Could you check a few things on this model? Use its own coordinates, in mm. A direction names the side the tool comes from. Round coordinates to 2 decimals unless told otherwise and drop trailing zeros. Loops run counter-clockwise (first coordinate to the right, second up) from the corner with the lowest first, then second, coordinate; pieces in that order, holes last. Notation, with made-up numbers: (-37, 87) - (19, 87) arc R14 ccw to (19, 97) - close; hole circle Ø3 at (-18, 61). An arc over 180 degrees is marked (long way). Answer as CSV lines item,"result". Start each with the question number.
1) Suppose I cut it at B-B, the plane z = 13.5. Write out the boundary of the cut face in (x, y), then the cut area to 3 significant figures.
2) We'd pull the mould along Z, two halves only. Please class faces 1 (the face through (61, 20, 26.5)), 2 (the face through (15.175, 68.335, 22.204)), 3 (the face through (66.94, 0.09, 5.8)): pulls with the +Z half, pulls with the -Z half, needs draft (parallel to the pull), parting line crosses it, or undercut.
3) Which directions (+Z, -Z, +X, -X, +Y, -Y) give clear straight access to the entire face, cutting with the end or side of a thin tool? Please do faces 4 (the face through (52, 46, 9)), 5 (the face through (15.175, 68.335, 5.704)).
4) Please list where these lines run through material, in increasing order: line 1 along Z through (x, y) = (31, -62); line 2 along Y through (x, z) = (0, 12.5); line 3 along Y through (x, z) = (-14.5, 7).
5) Suppose I cut it at A-A, the plane x = 0. Write out the boundary of the cut face in (y, z), then the cut area to 3 significant figures.
6) I'm going to push flat-ended pins straight in: pin 1 Ø6 at (y, z) = (54.5, 7.5) entering from -X; pin 2 Ø1 at (y, z) = (50, 9) entering from +X; pin 3 Ø12 at (x, z) = (-53, 14.5) entering from -Y. Where does each tip first touch, or does it pass through?
```python
from build123d import *

# Parameters (mm, degrees)
SKETCH2_R           = 2.2
GRUB_KEY_HOLE_DEPTH = 8


with BuildPart() as part:
    # Sketch1 → Tyre (revolve)
    with BuildSketch(Plane(origin=(0, 0, 0), x_dir=(0, 0, -1), z_dir=(1, 0, 0)), mode=Mode.PRIVATE) as tyre_sk:
        Polygon((-1.5, 64), (-26.5, 64), (-26.5, 69), (-25.5, 70), (-19, 70), (-19, 68.8), (-17, 68.8), (-17, 70), (-11, 70), (-11, 68.8), (-9, 68.8), (-9, 70), (-2.5, 70), (-1.5, 69), align=None)
    revolve(tyre_sk.sketch.rotate(Axis((0, 0, 0), (0, 0, 1)), 90), axis=Axis((0, 0, 0), (0, 0, 1)))

    # Sketch2 → Grub_key_hole (cut)
    with BuildSketch(Plane(origin=(63, 0, 0), x_dir=(0, 0, -1), z_dir=(1, 0, 0))):
        with Locations((-3.6, 0)):
            Circle(SKETCH2_R)
    extrude(amount=GRUB_KEY_HOLE_DEPTH, mode=Mode.SUBTRACT)


solid = part.part
```
Filled sheet:
1,outline,"circle Ø140 at (0, 0); hole circle Ø128 at (0, 0)"
1,area,"2,530 mm²"
2,face 1,"pulls with the +Z half"
2,face 2,"needs draft"
2,face 3,"undercut"
3,face 4,"none"
3,face 5,"+Z, -Z"
4,line 1,"1.82 to 9, 11 to 17, 19 to 26.18"
4,line 2,"-70 to -64, 64 to 70"
4,line 3,"-68.48 to -62.34, 62.34 to 68.48"
5,outline,"(-70, 2.5) - (-69, 1.5) - (-64, 1.5) - (-64, 26.5) - (-69, 26.5) - (-70, 25.5) - (-70, 19) - (-68.8, 19) - (-68.8, 17) - (-70, 17) - (-70, 11) - (-68.8, 11) - (-68.8, 9) - (-70, 9) - close; (64, 1.5) - (69, 1.5) - (70, 2.5) - (70, 9) - (68.8, 9) - (68.8, 11) - (70, 11) - (70, 17) - (68.8, 17) - (68.8, 19) - (70, 19) - (70, 25.5) - (69, 26.5) - (64, 26.5) - close"
5,area,"288 mm²"
6,pin 1,"x = -47.41"
6,pin 2,"x = 49.49"
6,pin 3,"y = -51.87"
